```python
from build123d import *

# Parameters (mm, degrees)
F0_W        = 57
F0_H        = 57
F0_R        = 25
F1_DEPTH    = 25
F2_T1_DEPTH = 175
F3_R        = 20


# Not quite as in the source:
# - a fillet or chamfer that OpenCascade refuses, or shapes differently, is made with other operations: its cross-section is extruded or revolved along the edge and cut away or added


with BuildPart() as f1:
    # F0 (on Front) → F1 (new body)
    with BuildSketch(Plane.XZ):
        Rectangle(F0_W, F0_H)
        Circle(F0_R, mode=Mode.SUBTRACT)
    extrude(amount=F1_DEPTH)

    # F2: fillet of radius 30 on 2 edges, made by hand

    # F2_s2 → F2_t1 (cut)
    with BuildSketch(Plane.XZ.offset(-75)):
        with BuildLine():
            ThreePointArc((28.5, -1.5), (19.7132034356, 19.7132034356), (-1.5, 28.5))
            Line((-1.5, 28.5), (28.5, 28.5))
            Line((28.5, 28.5), (28.5, -1.5))
        make_face()
        with BuildLine():
            ThreePointArc((1.5, 28.5), (-19.7132034356, 19.7132034356), (-28.5, -1.5))
            Line((-28.5, -1.5), (-28.5, 28.5))
            Line((-28.5, 28.5), (1.5, 28.5))
        make_face()
    extrude(amount=F2_T1_DEPTH, mode=Mode.SUBTRACT)

    # F3
    f3_edges = [f1.edges().sort_by_distance(p)[0] for p in [
        (0, -12.5, 28.462477),
    ]]
    fillet(f3_edges, radius=F3_R)


solid = f1.part
```
CAD build for the part. Positions are in the model's coordinates, mm. Coordinates: 2 decimals unless noted, no trailing zeros. Order: outer loops, then holes, each group sorted by start corner. A loop starts at its lowest first (then second) coordinate and runs counter-clockwise, first axis right, second up. Notation, with made-up numbers: M -21,-22 L -8,-22 A18 cw -8,12 Z; hole C 49,-23 d4. An arc over 180 degrees is marked long. Write each question's results on one line, items separated by ' | '. Start each with the question number.
Q1. Cut at A-A (x = 11.5). List the corners of the cut face in (y, z).
Q2. Pull direction Z, two halves, no side cores. Call faces 1 (the flat face through (0, -12, -28.5)), 2 (the cylindrical face through (23.846, -12.325, 7.509)), 3 (the flat face through (28.5, -12, -15)), 4 (the cylindrical face through (21.44, -12.33, 17.83)): +Z half, -Z half, draft (parallel to the pull), parting line (faces both ways), or undercut.
Q3. Drill centre lines: probe 1 along Z at (x, y) = (0, -15.75); probe 2 along Z at (x, y) = (13.5, -18.75); probe 3 along X at (y, z) = (-2, -3.5). Where is each one in solid material? Low to high. Write a range as from..to.
Q4. Cut at B-B (z = 0). List the corners of the cut face in (x, y).
Q5. Flat gauge pins, fed straight in: P1, Ø2, axis at x = 16, y = -10, coming from the +Z side; P2, Ø12, axis at x = 16, y = -17, coming from the +Z side; P3, Ø10, axis at y = -9.5, z = 4.5, coming from the -X side. Where does each tip first touch, or does it go through?
Found:
1) outline: M -25,-28.5 L 0,-28.5 L 0,-22.2 L -25,-22.2 Z; M -25,22.2 L 0,22.2 L 0,25.54 L -25,25.54 Z
2) face 1: -Z half | face 2: undercut | face 3: draft | face 4: +Z half
3) probe 1: -28.5..-25, 25..28.39 | probe 2: -28.5..-21.04, 21.04..24.48 | probe 3: -28.5..-24.75, 24.75..28.5
4) outline: M -28.46,-25 L -25,-25 L -25,0 L -28.46,0 Z; M 25,-25 L 28.46,-25 L 28.46,0 L 25,0 Z
5) P1: z = 23.55 | P2: z = 26.21 | P3: x = -28.48
